```python
from build123d import *

# Parameters (mm, degrees)
SKETCH1_W               = 300
SKETCH1_H               = 170
BOSS_EXTRUDE1_DEPTH     = 10
SKETCH2_W               = 290
SKETCH2_H               = 160
SKETCH2_W_2             = 286
SKETCH2_H_2             = 156
CUT_EXTRUDE1_DEPTH      = 5
SKETCH5_W               = 286
SKETCH5_H               = 156
CUT_EXTRUDE2_DEPTH      = 28
CUT_EXTRUDE2_DEPTH_BACK = 40


with BuildPart() as part:
    # Sketch1 → Boss-Extrude1 (new body)
    with BuildSketch(Plane(origin=(0, 0, 0), x_dir=(1, 0, 0), z_dir=(0, 1, 0))):
        with Locations((-10.575275385, -12.987279515)):
            Rectangle(SKETCH1_W, SKETCH1_H)
    extrude(amount=BOSS_EXTRUDE1_DEPTH)

    # Sketch2 → Cut-Extrude1 (cut)
    with BuildSketch(Plane(origin=(0, 10, 0), x_dir=(1, 0, 0), z_dir=(0, 1, 0))):
        with Locations((-10.575275385, -12.987279515)):
            Rectangle(SKETCH2_W, SKETCH2_H)
        with Locations((-10.575275385, -12.987279515)):
            Rectangle(SKETCH2_W_2, SKETCH2_H_2, mode=Mode.SUBTRACT)
    extrude(amount=-CUT_EXTRUDE1_DEPTH, mode=Mode.SUBTRACT)

    # Sketch5 → Cut-Extrude2 (cut, two sides)
    with BuildSketch(Plane(origin=(0, 10, 0), x_dir=(1, 0, 0), z_dir=(0, 1, 0))) as cut_extrude2_sk:
        with Locations((-10.575275385, -12.987279515)):
            Rectangle(SKETCH5_W, SKETCH5_H)
    extrude(amount=CUT_EXTRUDE2_DEPTH, mode=Mode.SUBTRACT)
    extrude(cut_extrude2_sk.sketch, amount=-CUT_EXTRUDE2_DEPTH_BACK, mode=Mode.SUBTRACT)


solid = part.part
```
Check sheet for the modelled part. Datum: model origin and axes. Units: mm. Coordinates: 2 decimals unless noted, no trailing zeros. Write each loop counter-clockwise with the first axis right and the second up, starting at its lowest first coordinate (ties: lowest second). Pieces come first, ordered by that corner, then holes. Notation, with made-up numbers: M 14,67 L 33,67 A25 ccw 33,90 Z; hole C 39,58 d2. An arc over 180 degrees is marked long. Write item = value, one per line. Start each with the question number.
1. Sectioned sample at C-C (y = 7.75). Record the cut outline in (x, z).
2. Mould release check, pull along X, two halves, no side actions. Record for faces 1 (the flat face through (-56, 10, -69)), 2 (the flat face through (-160.575, 5, 14)), 3 (the flat face through (139.425, 5, 14)): pulls with the +X half, pulls with the -X half, needs draft (parallel to the pull), parting line crosses it, or undercut.
3. Sectioned sample at B-B (x = -138.5). Record the cut outline in (y, z), then the cut area to 3 significant figures.
4. Thickness scan on probe 1 along Z at (x, y) = (-82, 1.5); probe 2 along Z at (x, y) = (41.5, 8.25); probe 3 along X at (y, z) = (3.75, 23.5). Record the ranges inside material, lowest first.
5. Sectioned sample at A-A (z = 31). Record the cut outline in (x, y).
The answers:
q1.outline = M -160.58,-72.01 L 139.42,-72.01 L 139.42,97.99 L -160.58,97.99 Z; hole M -155.58,-67.01 L 134.42,-67.01 L 134.42,92.99 L -155.58,92.99 Z
q2.face_1 = needs draft
q2.face_2 = pulls with the -X half
q2.face_3 = pulls with the +X half
q3.outline = M 0,-72.01 L 10,-72.01 L 10,-67.01 L 5,-67.01 L 5,-65.01 L 0,-65.01 Z; M 0,90.99 L 5,90.99 L 5,92.99 L 10,92.99 L 10,97.99 L 0,97.99 Z
q3.area = 120 mm²
q4.probe_1 = -72.01 to -65.01, 90.99 to 97.99
q4.probe_2 = -72.01 to -67.01, 92.99 to 97.99
q4.probe_3 = -160.58 to -153.58, 132.42 to 139.42
q5.outline = M -160.58,0 L -153.58,0 L -153.58,5 L -155.58,5 L -155.58,10 L -160.58,10 Z; M 132.42,0 L 139.42,0 L 139.42,10 L 134.42,10 L 134.42,5 L 132.42,5 Z
